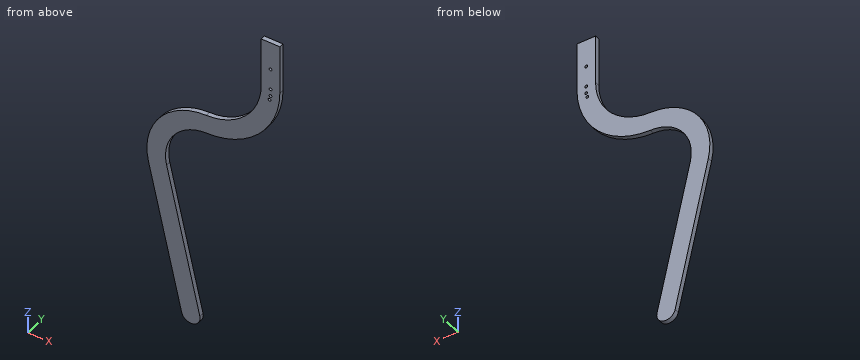
```python
from build123d import *

# Parameters (mm, degrees)
SKETCH_1_R          = 1.5
EXTRUDE_1_DEPTH     = 5
SKETCH_2_R          = 1.5
CUT_EXTRUDE_2_DEPTH = 195.128306699


with BuildPart() as part:
    # 草圖1 → 伸長1 (new body)
    with BuildSketch(Plane(origin=(0, 0, 0), x_dir=(1, 0, 0), z_dir=(0, 1, 0))):
        with BuildLine():
            Line((57.897360436, -125.299605011), (57.897360436, -177.743637577))
            Line((57.897360436, -177.743637577), (77.897360436, -177.743637577))
            Line((77.897360436, -177.743637577), (77.897360436, -125.299605011))
            ThreePointArc((77.897360436, -125.299605011), (54.918314005, -69.05496851), (-0.871008877, -44.991569694))
            ThreePointArc((-0.871008877, -44.991569694), (-35.489867026, -27.667116556), (-43.844435656, 10.132396657))
            Line((-43.844435656, 10.132396657), (-8.109110739, 164.764632944))
            ThreePointArc((-8.109110739, 164.764632944), (-15.600674961, 176.759484569), (-27.595526586, 169.267920347))
            Line((-27.595526586, 169.267920347), (-63.330851503, 14.63568406))
            ThreePointArc((-63.330851503, 14.63568406), (-51.263141259, -39.963612803), (-1.258123933, -64.987822891))
            ThreePointArc((-1.258123933, -64.987822891), (40.639968493, -83.059569519), (57.897360436, -125.299605011))
        make_face()
        with Locations(Location((66.82899479, -113.088129791, 0), (0, 0, 270))):
            Circle(SKETCH_1_R, mode=Mode.SUBTRACT)
        with Locations(Location((67.897360436, -125.299605011, 0), (0, 0, 270))):
            Circle(SKETCH_1_R, mode=Mode.SUBTRACT)
    extrude(amount=EXTRUDE_1_DEPTH)

    # 草圖2 → 伸長2 (cut, through all)
    with BuildSketch(Plane(origin=(0, 5, 0), x_dir=(1, 0, 0), z_dir=(0, 1, 0))):
        with Locations(Location((67.897360436, -117.743637577, 0), (0, 0, 270))):
            Circle(SKETCH_2_R)
        with Locations(Location((67.897360436, -147.743637577, 0), (0, 0, 270))):
            Circle(SKETCH_2_R)
    extrude(amount=-CUT_EXTRUDE_2_DEPTH, mode=Mode.SUBTRACT)


solid = part.part
```
Could you check a few things on this model? Use its own coordinates, in mm. Round coordinates to 2 decimals unless told otherwise and drop trailing zeros. Loops run counter-clockwise (first coordinate to the right, second up) from the corner with the lowest first, then second, coordinate; pieces in that order, holes last. Notation, with made-up numbers: M 74,5.5 L 132,5.5 A21 cw 132,42.5 Z; hole C -29.5,33.5 d2. An arc over 180 degrees is marked long. Write item = value, one per line.
1. I want a section at D-D, the plane x = 49. Write out the boundary of the cut face in (y, z), and give its area (3 significant figures).
Results below:
outline = M 0,63.6 L 5,63.6 L 5,93.77 L 0,93.77 Z
area = 151 mm²
2. I want a section at C-C, the plane z = 138. Write out the boundary of the cut face in (x, y).
Results below:
outline = M 57.9,0 L 77.9,0 L 77.9,5 L 57.9,5 Z
3. I need wall thicknesses on probe 1 along X at (y, z) = (3, 136.5); probe 2 along X at (y, z) = (1.45, 32); probe 3 along Z at (x, y) = (37.5, 0.75). Which ranges of each line are inside material? Lowest first, please.
Results below:
probe_1 = 57.9 to 77.9
probe_2 = -56.58 to -31.64
probe_3 = 55.6 to 80.08
4. I want a section at B-B, the plane x = -36. Write out the boundary of the cut face in (y, z), and give its area (3 significant figures).
Results below:
outline = M 0,-132.9 L 5,-132.9 L 5,-44.08 L 0,-44.08 Z; M 0,27 L 5,27 L 5,54.12 L 0,54.12 Z
area = 580 mm²
5. I want a section at A-A, the plane y = 3.2. Write out the boundary of the cut face in (x, z), and give its area (3 significant figures).
Results below:
outline = M -63.33,-14.64 L -27.6,-169.27 A10 ccw -8.11,-164.76 L -43.84,-10.13 A45 cw -0.87,44.99 A80.32 ccw 77.9,125.3 L 77.9,177.74 L 57.9,177.74 L 57.9,125.3 A60.32 cw -1.26,64.99 A65 ccw Z; hole C 66.83,113.09 d3; hole C 67.9,117.74 d3; hole C 67.9,125.3 d3; hole C 67.9,147.74 d3
area = 8,490 mm²
